Read the model definition and answer for the solid it produces. Units are mm, in the model's axes. A direction names the side the tool comes from. Round coordinates to 2 decimals unless told otherwise and drop trailing zeros. Order: outer loops, then holes, each group sorted by start corner. A loop starts at its lowest first (then second) coordinate and runs counter-clockwise, first axis right, second up.
from build123d import *

# Parameters (mm, degrees)
SKETCH1_W                = 187
SKETCH1_H                = 112
SKETCH1_R                = 1.425
SKETCH1_W_2              = 176.5
SKETCH1_H_2              = 101.5
EDGE_2_DEPTH             = 16.1
SKETCH2_W                = 176.5
SKETCH2_H                = 101.5
TOP_COVER_DEPTH          = 3
COMPONENTS_CUTOUTS_REACH = 112.17
SKETCH3_W                = 12
SKETCH3_H                = 38
SKETCH3_W_2              = 13
SKETCH3_H_2              = 25
SKETCH3_W_3              = 25
SKETCH3_H_3              = 14
FAN_HOLES_REACH          = 112.17
SKETCH6_R                = 1.9
SKETCH6_R_2              = 18.5
SKETCH6_R_3              = 27.5
SKETCH4_W                = 155
SKETCH4_H                = 11.1
LENGTH_AIR_VENTS_DEPTH   = 147.783718443
SKETCH5_W                = 80
SKETCH5_H                = 11.1
WIDTH_AIR_VENTS_DEPTH    = 196.867838095
FILLET1_R                = 1


with BuildPart() as part:
    # Sketch1 → Edge 2 (new body)
    with BuildSketch(Plane(origin=(0, 0, 0), x_dir=(1, 0, 0), z_dir=(0, 1, 0))):
        Rectangle(SKETCH1_W, SKETCH1_H)
        with Locations(Location((-89.5, -52, 0), (0, 0, 270))):
            Circle(SKETCH1_R, mode=Mode.SUBTRACT)
        with Locations(Location((89.5, -52, 0), (0, 0, 270))):
            Circle(SKETCH1_R, mode=Mode.SUBTRACT)
        with Locations(Location((89.5, 52, 0), (0, 0, 270))):
            Circle(SKETCH1_R, mode=Mode.SUBTRACT)
        with Locations(Location((-89.5, 52, 0), (0, 0, 270))):
            Circle(SKETCH1_R, mode=Mode.SUBTRACT)
        Rectangle(SKETCH1_W_2, SKETCH1_H_2, mode=Mode.SUBTRACT)
    extrude(amount=EDGE_2_DEPTH)

    # Sketch2 → Top Cover (add)
    with BuildSketch(Plane(origin=(0, 16.1, 0), x_dir=(1, 0, 0), z_dir=(0, 1, 0))):
        Rectangle(SKETCH2_W, SKETCH2_H)
    extrude(amount=-TOP_COVER_DEPTH)

    # Sketch3 → Components Cutouts (cut, up to next)
    with BuildSketch(Plane(origin=(0, 16.1, 0), x_dir=(1, 0, 0), z_dir=(0, 1, 0)), mode=Mode.PRIVATE) as components_cutouts_sk1:
        with Locations((-81.5, -23)):
            Rectangle(SKETCH3_W, SKETCH3_H)
    components_cutouts_tool1 = extrude(components_cutouts_sk1.sketch, amount=-COMPONENTS_CUTOUTS_REACH, mode=Mode.PRIVATE) & part.part
    # Sketch3 → Components Cutouts (cut, up to next)
    with BuildSketch(Plane(origin=(0, 16.1, 0), x_dir=(1, 0, 0), z_dir=(0, 1, 0)), mode=Mode.PRIVATE) as components_cutouts_sk2:
        Polygon((-29.5, 36), (-29.5, -2), (14.5, -2), (14.5, 36.5), (-21, 36.5), (-21, 50), (-46, 50), (-46, 36), align=None)
    components_cutouts_tool2 = extrude(components_cutouts_sk2.sketch, amount=-COMPONENTS_CUTOUTS_REACH, mode=Mode.PRIVATE) & part.part
    # Sketch3 → Components Cutouts (cut, up to next)
    with BuildSketch(Plane(origin=(0, 16.1, 0), x_dir=(1, 0, 0), z_dir=(0, 1, 0)), mode=Mode.PRIVATE) as components_cutouts_sk3:
        with Locations((-81, 22.5)):
            Rectangle(SKETCH3_W_2, SKETCH3_H_2)
    components_cutouts_tool3 = extrude(components_cutouts_sk3.sketch, amount=-COMPONENTS_CUTOUTS_REACH, mode=Mode.PRIVATE) & part.part
    # Sketch3 → Components Cutouts (cut, up to next)
    with BuildSketch(Plane(origin=(0, 16.1, 0), x_dir=(1, 0, 0), z_dir=(0, 1, 0)), mode=Mode.PRIVATE) as components_cutouts_sk4:
        Polygon((60, -38.5), (60, -37), (74, -37), (74, 28), (87.5, 28), (87.5, -39), (78.5, -39), (78.5, -50), (-74, -50), (-74, -38.5), align=None)
    components_cutouts_tool4 = extrude(components_cutouts_sk4.sketch, amount=-COMPONENTS_CUTOUTS_REACH, mode=Mode.PRIVATE) & part.part
    # Sketch3 → Components Cutouts (cut, up to next)
    with BuildSketch(Plane(origin=(0, 16.1, 0), x_dir=(1, 0, 0), z_dir=(0, 1, 0)), mode=Mode.PRIVATE) as components_cutouts_sk5:
        with Locations((28.5, 43)):
            Rectangle(SKETCH3_W_3, SKETCH3_H_3)
    components_cutouts_tool5 = extrude(components_cutouts_sk5.sketch, amount=-COMPONENTS_CUTOUTS_REACH, mode=Mode.PRIVATE) & part.part
    add(components_cutouts_tool1.solids().sort_by_distance((-81.5, 16.1, 23))[0], mode=Mode.SUBTRACT)
    add(components_cutouts_tool2.solids().sort_by_distance((-11.924347, 16.1, -21.628845))[0], mode=Mode.SUBTRACT)
    add(components_cutouts_tool3.solids().sort_by_distance((-81, 16.1, -22.5))[0], mode=Mode.SUBTRACT)
    add(components_cutouts_tool4.solids().sort_by_distance((61.793495, 16.1, 37.75))[0], mode=Mode.SUBTRACT)
    add(components_cutouts_tool5.solids().sort_by_distance((28.5, 16.1, -43))[0], mode=Mode.SUBTRACT)

    # Sketch6 → Fan Holes (cut, up to next)
    with BuildSketch(Plane(origin=(0, 16.1, 0), x_dir=(1, 0, 0), z_dir=(0, 1, 0)), mode=Mode.PRIVATE) as fan_holes_sk1:
        with Locations(Location((-65.5, -4, 0), (0, 0, 270))):
            Circle(SKETCH6_R)
    fan_holes_tool1 = extrude(fan_holes_sk1.sketch, amount=-FAN_HOLES_REACH, mode=Mode.PRIVATE) & part.part
    # Sketch6 → Fan Holes (cut, up to next)
    with BuildSketch(Plane(origin=(0, 16.1, 0), x_dir=(1, 0, 0), z_dir=(0, 1, 0)), mode=Mode.PRIVATE) as fan_holes_sk2:
        with Locations(Location((-65.5, 28, 0), (0, 0, 270))):
            Circle(SKETCH6_R)
    fan_holes_tool2 = extrude(fan_holes_sk2.sketch, amount=-FAN_HOLES_REACH, mode=Mode.PRIVATE) & part.part
    # Sketch6 → Fan Holes (cut, up to next)
    with BuildSketch(Plane(origin=(0, 16.1, 0), x_dir=(1, 0, 0), z_dir=(0, 1, 0)), mode=Mode.PRIVATE) as fan_holes_sk3:
        with Locations(Location((-33.5, 28, 0), (0, 0, 270))):
            Circle(SKETCH6_R)
    fan_holes_tool3 = extrude(fan_holes_sk3.sketch, amount=-FAN_HOLES_REACH, mode=Mode.PRIVATE) & part.part
    # Sketch6 → Fan Holes (cut, up to next)
    with BuildSketch(Plane(origin=(0, 16.1, 0), x_dir=(1, 0, 0), z_dir=(0, 1, 0)), mode=Mode.PRIVATE) as fan_holes_sk4:
        with Locations(Location((-33.5, -4, 0), (0, 0, 270))):
            Circle(SKETCH6_R)
    fan_holes_tool4 = extrude(fan_holes_sk4.sketch, amount=-FAN_HOLES_REACH, mode=Mode.PRIVATE) & part.part
    # Sketch6 → Fan Holes (cut, up to next)
    with BuildSketch(Plane(origin=(0, 16.1, 0), x_dir=(1, 0, 0), z_dir=(0, 1, 0)), mode=Mode.PRIVATE) as fan_holes_sk5:
        with Locations(Location((-49.5, 12, 0), (0, 0, 270))):
            Circle(SKETCH6_R_2)
    fan_holes_tool5 = extrude(fan_holes_sk5.sketch, amount=-FAN_HOLES_REACH, mode=Mode.PRIVATE) & part.part
    # Sketch6 → Fan Holes (cut, up to next)
    with BuildSketch(Plane(origin=(0, 16.1, 0), x_dir=(1, 0, 0), z_dir=(0, 1, 0)), mode=Mode.PRIVATE) as fan_holes_sk6:
        with Locations(Location((44.5, 6, 0), (0, 0, 270))):
            Circle(SKETCH6_R_3)
    fan_holes_tool6 = extrude(fan_holes_sk6.sketch, amount=-FAN_HOLES_REACH, mode=Mode.PRIVATE) & part.part
    # Sketch6 → Fan Holes (cut, up to next)
    with BuildSketch(Plane(origin=(0, 16.1, 0), x_dir=(1, 0, 0), z_dir=(0, 1, 0)), mode=Mode.PRIVATE) as fan_holes_sk7:
        with Locations(Location((19.5, -19, 0), (0, 0, 270))):
            Circle(SKETCH6_R)
    fan_holes_tool7 = extrude(fan_holes_sk7.sketch, amount=-FAN_HOLES_REACH, mode=Mode.PRIVATE) & part.part
    # Sketch6 → Fan Holes (cut, up to next)
    with BuildSketch(Plane(origin=(0, 16.1, 0), x_dir=(1, 0, 0), z_dir=(0, 1, 0)), mode=Mode.PRIVATE) as fan_holes_sk8:
        with Locations(Location((69.5, -19, 0), (0, 0, 270))):
            Circle(SKETCH6_R)
    fan_holes_tool8 = extrude(fan_holes_sk8.sketch, amount=-FAN_HOLES_REACH, mode=Mode.PRIVATE) & part.part
    # Sketch6 → Fan Holes (cut, up to next)
    with BuildSketch(Plane(origin=(0, 16.1, 0), x_dir=(1, 0, 0), z_dir=(0, 1, 0)), mode=Mode.PRIVATE) as fan_holes_sk9:
        with Locations(Location((69.5, 31, 0), (0, 0, 270))):
            Circle(SKETCH6_R)
    fan_holes_tool9 = extrude(fan_holes_sk9.sketch, amount=-FAN_HOLES_REACH, mode=Mode.PRIVATE) & part.part
    # Sketch6 → Fan Holes (cut, up to next)
    with BuildSketch(Plane(origin=(0, 16.1, 0), x_dir=(1, 0, 0), z_dir=(0, 1, 0)), mode=Mode.PRIVATE) as fan_holes_sk10:
        with Locations(Location((19.5, 31, 0), (0, 0, 270))):
            Circle(SKETCH6_R)
    fan_holes_tool10 = extrude(fan_holes_sk10.sketch, amount=-FAN_HOLES_REACH, mode=Mode.PRIVATE) & part.part
    add(fan_holes_tool1.solids().sort_by_distance((-65.5, 16.1, 4))[0], mode=Mode.SUBTRACT)
    add(fan_holes_tool2.solids().sort_by_distance((-65.5, 16.1, -28))[0], mode=Mode.SUBTRACT)
    add(fan_holes_tool3.solids().sort_by_distance((-33.5, 16.1, -28))[0], mode=Mode.SUBTRACT)
    add(fan_holes_tool4.solids().sort_by_distance((-33.5, 16.1, 4))[0], mode=Mode.SUBTRACT)
    add(fan_holes_tool5.solids().sort_by_distance((-49.5, 16.1, -12))[0], mode=Mode.SUBTRACT)
    add(fan_holes_tool6.solids().sort_by_distance((44.5, 16.1, -6))[0], mode=Mode.SUBTRACT)
    add(fan_holes_tool7.solids().sort_by_distance((19.5, 16.1, 19))[0], mode=Mode.SUBTRACT)
    add(fan_holes_tool8.solids().sort_by_distance((69.5, 16.1, 19))[0], mode=Mode.SUBTRACT)
    add(fan_holes_tool9.solids().sort_by_distance((69.5, 16.1, -31))[0], mode=Mode.SUBTRACT)
    add(fan_holes_tool10.solids().sort_by_distance((19.5, 16.1, -31))[0], mode=Mode.SUBTRACT)

    # Sketch4 → Length Air Vents (cut, through all)
    with BuildSketch(Plane.XY.offset(56)):
        with Locations((0, 5.55)):
            Rectangle(SKETCH4_W, SKETCH4_H)
    extrude(amount=-LENGTH_AIR_VENTS_DEPTH, mode=Mode.SUBTRACT)

    # Sketch5 → Width Air Vents (cut, through all)
    with BuildSketch(Plane.ZY.offset(93.5)):
        with Locations((0, 5.55)):
            Rectangle(SKETCH5_W, SKETCH5_H)
    extrude(amount=-WIDTH_AIR_VENTS_DEPTH, mode=Mode.SUBTRACT)

    # Fillet1
    fillet1_edges = [part.edges().sort_by_distance(p)[0] for p in [
        (93.5, 16.1, 0),
        (0, 16.1, -56),
        (-93.5, 16.1, 0),
        (-93.5, 8.05, -56),
        (93.5, 8.05, -56),
        (93.5, 8.05, 56),
        (-93.5, 8.05, 56),
        (0, 16.1, 56),
    ]]
    fillet(fillet1_edges, radius=FILLET1_R)


solid = part.part
Q1. For a pull along X with two mould halves and no side action, classify faces 1 (the face through (-93.5, 12, 1)), 2 (the face through (0, 12, -50.75)), 3 (the face through (-67.56, 14.62, -16.01)), 4 (the face through (-91, 11.1, -1)) as released by +X, released by -X, zero draft, split by the parting line, or undercut.
Outcome:
face 1: released by -X
face 2: undercut
face 3: undercut
face 4: zero draft
Q2. A cutting plane is placed at A-A, the plane y = 6. Give the number of separate pieces and of enclosed holes in the cut face, plus the area to 3 significant figures.
Outcome:
separate pieces: 4
enclosed holes: 4
area: 535 mm2
Q3. A cutting plane is placed at B-B, the plane z = 45. Give the vertices of the cut face in (x, y).
Outcome:
outline: (-93.5, 0) - (-88.25, 0) - (-88.25, 13.1) - (-74, 13.1) - (-74, 16.1) - (-92.5, 16.1) arc R1 ccw to (-93.5, 15.1) - close; (78.5, 13.1) - (88.25, 13.1) - (88.25, 0) - (93.5, 0) - (93.5, 15.1) arc R1 ccw to (92.5, 16.1) - (78.5, 16.1) - close
Q4. Straight lines are drawn through the part: probe 1 along Z at (x, y) = (89.5, 7.75) (3 decimals); probe 2 along X at (y, z) = (6.75, 52) (3 decimals); probe 3 along X at (y, z) = (11.5, 18). For each, find the intervals that lie inside material, in ascending order.
Outcome:
probe 1: z = -56 to -53.425, -50.575 to -40, 40 to 50.575, 53.425 to 56
probe 2: x = -93.5 to -90.925, -88.075 to -77.5, 77.5 to 88.075, 90.925 to 93.5
probe 3: x = -93.5 to -88.25, 88.25 to 93.5
Q5. A flat-ended cylindrical pin translates along its axis: pin 1 (2.5 mm diameter, centred on x = -90.5, z = 18, fed in from -Y). Find the tip coordinate at first contact, or state that the pin passes through.
Outcome:
pin 1: stops at y = 11.1
Q6. A cutting plane is placed at C-C, the plane x = 7. Give the vertices of the cut face in (y, z), plus the area to 3 significant figures.
Outcome:
outline: (11.1, -56) - (15.1, -56) arc R1 ccw to (16.1, -55) - (16.1, -36.5) - (13.1, -36.5) - (13.1, -50.75) - (11.1, -50.75) - close; (11.1, 50.75) - (13.1, 50.75) - (13.1, 50) - (16.1, 50) - (16.1, 55) arc R1 ccw to (15.1, 56) - (11.1, 56) - close; (13.1, 2) - (16.1, 2) - (16.1, 38.5) - (13.1, 38.5) - close
area: 207 mm2
Q7. A cutting plane is placed at D-D, the plane x = 69.5. Give the vertices of the cut face in (y, z), plus the area to 3 significant figures.
Outcome:
outline: (11.1, -56) - (15.1, -56) arc R1 ccw to (16.1, -55) - (16.1, -32.9) - (13.1, -32.9) - (13.1, -50.75) - (11.1, -50.75) - close; (11.1, 50.75) - (13.1, 50.75) - (13.1, 50) - (16.1, 50) - (16.1, 55) arc R1 ccw to (15.1, 56) - (11.1, 56) - close; (13.1, -29.1) - (16.1, -29.1) - (16.1, -17.46) - (13.1, -17.46) - close; (13.1, 5.46) - (16.1, 5.46) - (16.1, 17.1) - (13.1, 17.1) - close; (13.1, 20.9) - (16.1, 20.9) - (16.1, 37) - (13.1, 37) - close
area: 226 mm2
Q8. For faces 5 (the face through (-91, 5, -40)), 6 (the face through (77.5, 5, -53)), 7 (the face through (88.25, 12, 0)), determine the directions among +Z, -Z, +X, -X, +Y, -Y from which every point of the face is accessible in a straight line to the end or side of a thin tool.
Outcome:
face 5: +X, -X, -Y
face 6: +Z, -Z, -Y
face 7: -Y
